Answer from the drawing. Dimensions are ordinates in mm from the lowest x, y and z of the part. Round coordinates to 2 decimals unless told otherwise and drop trailing zeros. Loops run counter-clockwise (first coordinate to the right, second up) from the corner with the lowest first, then second, coordinate; pieces in that order, holes last. Notation, with made-up numbers: (20, 49.25) -> (27, 49.25) arc R19 cw to (27, 57.25) -> close; hole circle Ø4 at (54, 10.25). An arc over 180 degrees is marked (long way). Use CSV: the item, a comma, the result in double quotes. Start each with the question number.
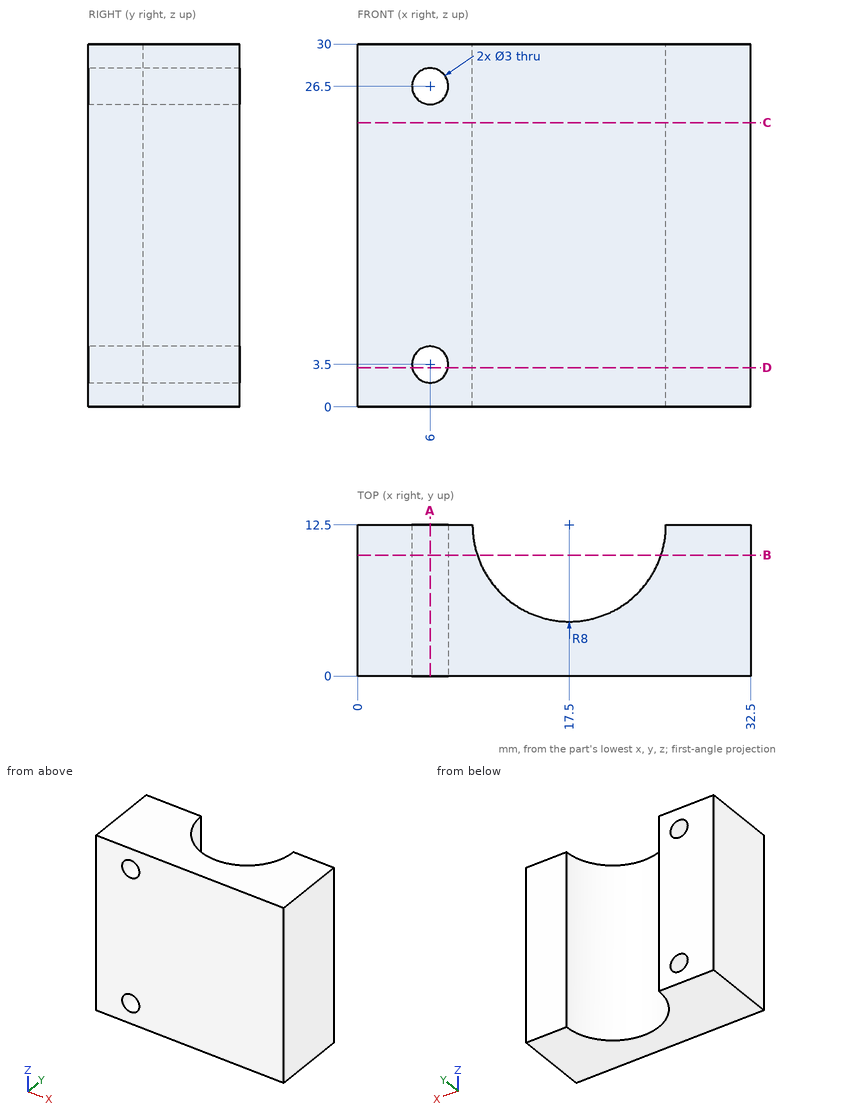
Q1. Section D-D, the plane z = 3.25 is taken. Write down the section's boundary in (x, y).
Q2. Straight lines are drawn through the part: line 1 (Z direction, x = 5, y = 10.75); line 2 (X direction, y = 6.25, z = 26.5); line 3 (X direction, y = 8.5, z = 26.5). For each, find the intervals that lie inside material, in ascending order. Write a range as from..to.
Q3. Each of these flat-tipped pins is pushed along its axis until it touches: pin 1 (12 mm diameter, centred on x = 17.5, z = 20.5, fed in from +Y); pin 2 (2.5 mm diameter, centred on x = 6, z = 3.5, fed in from +Y) (1 decimal). Where does it stop, or does it pass through?
Q4. Section C-C, the plane z = 23.5 is taken. Write down the section's boundary in (x, y).
Q5. Section B-B, the plane y = 10 is taken. Write down the section's boundary in (x, z).
Q6. Section A-A, the plane x = 6 is taken. Write down the section's boundary in (y, z), and give its area (3 significant figures).
Report:
1,outline,"(0, 0) -> (4.52, 0) -> (4.52, 12.5) -> (0, 12.5) -> close; (7.48, 0) -> (32.5, 0) -> (32.5, 12.5) -> (25.5, 12.5) arc R8 cw to (9.5, 12.5) -> (7.48, 12.5) -> close"
2,line 1,"z = 0..2.38, 4.62..25.38, 27.62..30"
2,line 2,"x = 0..4.5, 7.5..12.51, 22.49..32.5"
2,line 3,"x = 0..4.5, 7.5..10.57, 24.43..32.5"
3,pin 1,"stops at y = 7.21"
3,pin 2,"passes through"
4,outline,"(0, 0) -> (32.5, 0) -> (32.5, 12.5) -> (25.5, 12.5) arc R8 cw to (9.5, 12.5) -> (0, 12.5) -> close"
5,outline,"(0, 0) -> (9.9, 0) -> (9.9, 30) -> (0, 30) -> close; (25.1, 0) -> (32.5, 0) -> (32.5, 30) -> (25.1, 30) -> close; hole circle Ø3 at (6, 3.5); hole circle Ø3 at (6, 26.5)"
6,outline,"(0, 0) -> (12.5, 0) -> (12.5, 2) -> (0, 2) -> close; (0, 5) -> (12.5, 5) -> (12.5, 25) -> (0, 25) -> close; (0, 28) -> (12.5, 28) -> (12.5, 30) -> (0, 30) -> close"
6,area,"300 mm²"
